Design review of the part built by this model. Coordinates are the model's own, in mm. A direction names the side the tool comes from. Round coordinates to 2 decimals unless told otherwise and drop trailing zeros. Loops run counter-clockwise (first coordinate to the right, second up) from the corner with the lowest first, then second, coordinate; pieces in that order, holes last. Notation, with made-up numbers: (33, -7.75) -> (89, -7.75) arc R25 cw to (89, 18.25) -> close; hole circle Ø3 at (63.25, 51.25). An arc over 180 degrees is marked (long way). Use a Markdown table: item, result. Add a question column.
from build123d import *

# Parameters (mm, degrees)
SKETCH005_W             = 90.3
SKETCH005_H             = 78.3
PAD003_DEPTH            = 7
SKETCH006_R             = 2.5
POCKET002_DEPTH         = 7.001
SKETCH008_W             = 50
SKETCH008_H             = 50
PAD004_DEPTH            = 25
FILLET_R                = 8
SKETCH009_R             = 34
PAD005_DEPTH            = 7
SKETCH010_R             = 7.5
PAD006_DEPTH            = 20
BODY002_PLACEMENT_ANGLE = 90


with BuildPart() as part:
    # Sketch005 → Pad003 (new body)
    with BuildSketch(Plane.XY):
        Rectangle(SKETCH005_W, SKETCH005_H)
    extrude(amount=PAD003_DEPTH)

    # Sketch006 (on Face6 of Pad003) → Pocket002 (cut, through all)
    with BuildSketch(Plane.XY.offset(7)):
        with Locations((-37.5, 32.25)):
            Circle(SKETCH006_R)
        with Locations((-37.5, -32.25)):
            Circle(SKETCH006_R)
        with Locations((37.5, -32.25)):
            Circle(SKETCH006_R)
        with Locations((37.5, 32.25)):
            Circle(SKETCH006_R)
    extrude(amount=-POCKET002_DEPTH, mode=Mode.SUBTRACT)

    # Sketch007 → Revolution (revolve)
    with BuildSketch(Plane.XZ):
        with BuildLine():
            Line((7.5, 0), (7.5, 30))
            Line((7.5, 30), (16.65, 62.95))
            ThreePointArc((16.65, 62.95), (11.773328, 74.723328), (0, 79.6))
            Line((0, 0), (0, 79.6))
            Line((7.5, 0), (0, 0))
        make_face()
    revolve(axis=Axis((0, 0, 0), (0, 0, 1)))

    # Sketch008 → Pad004 (join)
    with BuildSketch(Plane.XY):
        Rectangle(SKETCH008_W, SKETCH008_H)
    extrude(amount=-PAD004_DEPTH)

    # Fillet
    fillet_edges = [part.edges().sort_by_distance(p)[0] for p in [
        (25, -25, -12.5),
        (-25, 25, -12.5),
        (-25, -25, -12.5),
        (25, 25, -12.5),
    ]]
    fillet(fillet_edges, radius=FILLET_R)

    # Sketch009 (on Face15 of Pad004) → Pad005 (join)
    with BuildSketch(Plane(origin=(0, 0, -25), x_dir=(1, 0, 0), z_dir=(0, 0, -1))):
        Circle(SKETCH009_R)
    extrude(amount=PAD005_DEPTH)

    # Sketch010 (on Face22 of Pad005) → Pad006 (join)
    with BuildSketch(Plane(origin=(0, 0, -32), x_dir=(1, 0, 0), z_dir=(0, 0, -1))):
        Circle(SKETCH010_R)
    extrude(amount=PAD006_DEPTH)


with BuildPart() as part_1:
    # Body002 placement: moved
    add(part.part.moved(Location((-130, 0, 480))).rotate(Axis((-130, 0, 480), (0, 0, 1)), BODY002_PLACEMENT_ANGLE))


solid = part_1.part
1. Mouldability with a two-part tool opening along Y and no side actions: class faces 4 (the face through (-99.86, -36.16, 483.55)), 5 (the face through (-129, 45.15, 483)), 6 (the face through (-107.281, -22.594, 467.325)) as +Y half, -Y half, draft (parallel to the pull), parting line (faces both ways), or undercut.
2. For faces 1 (the face through (-163.19, -7.37, 451.55)), 2 (the face through (-107.281, 22.594, 467.325)), 3 (the face through (-130, -25, 468)), list the 3-axis set-ups (+Z, -Z, +X, -X, +Y, -Y) from which the entire face can be reached by the end or side of a thin tool; tool diameter is ignored.
3. Consider section C-C on z = 456.5. State the section outline as (x, y) points, plus the area to 3 significant figures.
4. Consider section A-A on y = -37.5. State the section outline as (x, z) points.
5. To check wall thickness, follow probe 1 along X at (y, z) = (37.5, 484); probe 2 along Y at (x, z) = (-162, 484). State the ranges of each line that lie inside material, in increasing order. Write a range as from..to.
6. Insertion check: P1, Ø12.5, axis at x = -131.5, z = 473, coming from the -Y side; P2, Ø1.5, axis at x = -127, y = -19.5, coming from the -Z side; P3, Ø8, axis at x = -112, y = -1.5, coming from the +Z side. Each pin has a flat end and moves straight along its axis. Give the tip position at first contact, or say it passes through.
7. Consider section D-D on x = -158. State the section outline as (y, z) points.
8. Consider section B-B on x = -97.75. State the section outline as (y, z) points.
Verdict:
| question | item | result |
|---|---|---|
| 1 | face 4 | undercut |
| 1 | face 5 | +Y half |
| 1 | face 6 | -Y half |
| 2 | face 1 | -Z |
| 2 | face 2 | +X, +Y |
| 2 | face 3 | +X, -X, -Y |
| 3 | outline | (-155, -17) arc R8 ccw to (-147, -25) -> (-113, -25) arc R8 ccw to (-105, -17) -> (-105, 17) arc R8 ccw to (-113, 25) -> (-147, 25) arc R8 ccw to (-155, 17) -> close |
| 3 | area | 2,450 mm² |
| 4 | outline | (-169.15, 480) -> (-164.75, 480) -> (-164.75, 487) -> (-169.15, 487) -> close; (-159.75, 480) -> (-100.25, 480) -> (-100.25, 487) -> (-159.75, 487) -> close; (-95.25, 480) -> (-90.85, 480) -> (-90.85, 487) -> (-95.25, 487) -> close |
| 5 | probe 1 | x = -169.15..-164.75, -159.75..-100.25, -95.25..-90.85 |
| 5 | probe 2 | y = -45.15..-39.99, -35.01..35.01, 39.99..45.15 |
| 6 | P1 | stops at y = -25 |
| 6 | P2 | stops at z = 448 |
| 6 | P3 | stops at z = 551.86 |
| 7 | outline | (-45.15, 480) -> (45.15, 480) -> (45.15, 487) -> (-45.15, 487) -> close; (-19.29, 448) -> (19.29, 448) -> (19.29, 455) -> (-19.29, 455) -> close |
| 8 | outline | (-45.15, 480) -> (-40, 480) -> (-40, 487) -> (-45.15, 487) -> close; (-35, 480) -> (35, 480) -> (35, 487) -> (-35, 487) -> close; (-10.77, 448) -> (10.77, 448) -> (10.77, 455) -> (-10.77, 455) -> close; (40, 480) -> (45.15, 480) -> (45.15, 487) -> (40, 487) -> close |
